from build123d import *

# Parameters (mm, degrees)
F0_W     = 169.1423505545
F0_H     = 178.8771897554
F1_DEPTH = 10
F1_TAPER = -6
F3_D     = 6.35
F4_R     = 44.8702969829
F5_DEPTH = 60


with BuildPart() as f1:
    # F0 (on Front) → F1 (new body, symmetric)
    with BuildSketch(Plane.XZ):
        with Locations((43.3839261532, 70.992641151)):
            Rectangle(F0_W, F0_H)
    extrude(amount=F1_DEPTH, both=True, taper=F1_TAPER)

    # F3 (through all)
    with Locations(Plane.XZ.offset(10)):
        with Locations((48.48498106, 66.4365887642)):
            Hole(F3_D / 2)

    # F4 (on face) → F5 (join)
    with BuildSketch(Plane.XZ.offset(10)):
        with Locations((48.48498106, 66.4365887642)):
            Circle(F4_R)
    extrude(amount=F5_DEPTH)


solid = f1.part
Can you work these out from the model? Positions are in its coordinate system, mm. Give positions to 0.01 mm unless a question says otherwise; leave off trailing zeros. Order: outer loops, then holes, each group sorted by start corner. A loop starts at its lowest first (then second) coordinate and runs counter-clockwise, first axis right, second up. Notation, with made-up numbers: M -15.5,1.5 L 29.5,1.5 A22 cw 29.5,18.5 Z; hole C 35,51 d4. An arc over 180 degrees is marked long. Use one line per item in the form item = value.
Item 1: Thinking about a two-plate mould opening in X: for faces 1 (the cylindrical face through (89.934, -39.58, 49.251)), 2 (the flat face through (48, -10, 66)), 3 (the flat face through (2, -10, 70)), 4 (the cylindrical face through (46.778, 0.14, 69.114)), which applies, pulls with the +X half, pulls with the -X half, needs draft (parallel to the pull), parting line crosses it, or undercut?
Values follow:
face_1 = parting line crosses it
face_2 = undercut
face_3 = needs draft
face_4 = undercut
Item 2: If I drill on line 1 along Y through (x, z) = (31, 119.5); line 2 along Z through (x, y) = (30, -9.5); line 3 along Z through (x, y) = (26.5, -20), over which ranges is the centre line in solid material (lowest first)? Write a range as [from, to].
Values follow:
line_1 = [-10, 10]
line_2 = [-19.44, 161.43]
line_3 = [27.32, 105.55]
Item 3: Will these pins go through, and if not, where does the flat tip stop? pin 1 Ø3 at (x, y) = (62, -13.5) entering from -Z; pin 2 Ø6 at (y, z) = (-57.5, 85.5) entering from +X; pin 3 Ø6 at (x, y) = (46, -55.5) entering from +Z.
Values follow:
pin_1 = 23.2
pin_2 = 90.38
pin_3 = 111.31
Item 4: If we section it at A-A, the plane y = -61.5: Write out the boundary of the cut face in (x, z), and give its area (3 significant figures).
Values follow:
outline = C 48.48,66.44 d89.74
area = 6,330 mm^2
